```python
from build123d import *

# Parameters (mm, degrees)
F0_W           = 105.471175
F0_H           = 60.14101
F1_DEPTH       = 25.4
F2_SIZE        = 5.08
F3_R           = 5.08
F5_D           = 6.35
F5_CBORE_D     = 25.4
F5_CBORE_DEPTH = 6.35
F6_R           = 5.08


with BuildPart() as f1:
    # F0 (on Top) → F1 (new body)
    with BuildSketch(Plane.XY):
        with Locations((2.355178, -5.891924)):
            Rectangle(F0_W, F0_H)
    extrude(amount=F1_DEPTH)

    # F2
    f2_edges = [f1.edges().sort_by_distance(p)[0] for p in [
        (2.355179, -35.962429, 25.4),
    ]]
    chamfer(f2_edges, length=F2_SIZE)

    # F3
    f3_edges = [f1.edges().sort_by_distance(p)[0] for p in [
        (-50.380409, -3.351924, 25.4),
    ]]
    fillet(f3_edges, radius=F3_R)

    # F5 (through all)
    with Locations(Plane.YZ.offset(55.090766)):
        with Locations((-15.076851, 18.388513)):
            CounterBoreHole(F5_D / 2, F5_CBORE_D / 2, F5_CBORE_DEPTH)

    # F6
    f6_edges = [f1.edges().sort_by_distance(p)[0] for p in [
        (-50.380409, 24.178581, 10.16),
        (-48.892511, 24.178581, 23.912102),
        (2.355179, 24.178581, 0),
        (4.895179, 24.178581, 25.4),
        (55.090766, 24.178581, 12.7),
        (-50.380409, -5.891924, 0),
        (2.355179, -35.962429, 0),
        (55.090766, -5.891924, 0),
    ]]
    fillet(f6_edges, radius=F6_R)


solid = f1.part
```
Could you check a few things on this model? Use its own coordinates, in mm. A direction names the side the tool comes from. Round coordinates to 2 decimals unless told otherwise and drop trailing zeros. Loops run counter-clockwise (first coordinate to the right, second up) from the corner with the lowest first, then second, coordinate; pieces in that order, holes last. Notation, with made-up numbers: M 47.25,-36 L 103.25,-36 A32 cw 103.25,2 Z; hole C -16,1 d1. An arc over 180 degrees is marked long. Write item = value, one per line.
1. I want a section at D-D, the plane y = -32. Write out the boundary of the cut face in (x, z).
Results below:
outline = M -50.38,5.08 A5.08 ccw -46.42,0.12 L 51.13,0.12 A5.08 ccw 55.09,5.08 L 55.09,24.28 L -48.48,24.28 A5.08 ccw -50.38,20.32 Z
2. Thinking about a two-plate mould opening in Y: for faces 1 (the face through (51.96, -15.46, 5.694)), 2 (the face through (3.093, -34.435, 1.449)), 3 (the face through (-1.514, -14.664, 21.536)), 4 (the face through (-48.932, -8.046, 1.528)), which applies, +Y half, -Y half, draft (parallel to the pull), parting line (faces both ways), or undercut?
Results below:
face_1 = undercut
face_2 = -Y half
face_3 = undercut
face_4 = draft
3. Will this pin go through, and if not, where does the flat tip stop? P1, Ø6, axis at y = -11.5, z = 22, coming from the +X side.
Results below:
P1 = 48.74
4. I want a section at C-C, the plane z = 12.75. Write out the boundary of the cut face in (x, y), and give its area (3 significant figures).
Results below:
outline = M -50.38,-35.96 L 55.09,-35.96 L 55.09,-26.46 L 48.74,-26.46 L 48.74,-3.7 L 55.09,-3.7 L 55.09,19.1 A5.08 ccw 50.01,24.18 L -45.3,24.18 A5.08 ccw -50.38,19.1 Z
area = 6,190 mm²
5. I need wall thicknesses on probe 1 along Z at (x, y) = (2.5, -15); probe 2 along Y at (x, z) = (21, 18.75); probe 3 along Y at (x, z) = (16.5, 4.75). Which ranges of each line are inside material? Lowest first, please.
Results below:
probe_1 = 0 to 15.21, 21.56 to 25.4
probe_2 = -35.96 to -18.23, -11.92 to 24.18
probe_3 = -35.95 to 24.17
6. I want a section at A-A, the plane z = 17.25. Write out the boundary of the cut face in (x, y).
Results below:
outline = M -50.38,-35.96 L 55.09,-35.96 L 55.09,-27.73 L 48.74,-27.73 L 48.74,-18.04 L -50.38,-18.04 Z; M -50.38,-12.11 L 48.74,-12.11 L 48.74,-2.43 L 55.09,-2.43 L 55.09,19.1 A5.08 ccw 50.01,24.18 L -45.3,24.18 A5.08 ccw -50.38,19.1 Z
7. Which directions (+Z, -Z, +X, -X, +Y, -Y) give clear straight access to the entire face, cutting with the end or side of a thin tool? Please do faces 5 (the face through (48.741, -12, 16)), 6 (the face through (2, -6, 0)).
Results below:
face_5 = +X
face_6 = -Z, +X, -X, +Y, -Y
8. I want a section at B-B, the plane x = -18. Write out the boundary of the cut face in (y, z) (3 decimals), and give its area (3 significant figures).
Results below:
outline = M -35.962,5.08 A5.08 ccw -30.882,0 L 19.099,0 A5.08 ccw 24.179,5.08 L 24.179,20.32 A5.08 ccw 19.099,25.4 L -30.882,25.4 L -35.962,20.32 Z; hole C -15.077,18.389 d6.35
area = 1,470 mm²
